```python
from build123d import *

# Parameters (mm, degrees)
SKETCH1_R           = 24
SKETCH1_R_2         = 17.8
BOSS_EXTRUDE1_DEPTH = 3.05
SKETCH2_R           = 23.3
SKETCH2_R_2         = 19
CUT_EXTRUDE1_DEPTH  = 0.8
SKETCH3_R           = 22.7
SKETCH3_R_2         = 19.6
BOSS_EXTRUDE2_DEPTH = 2.3


with BuildPart() as part:
    # Sketch1 → Boss-Extrude1 (new, symmetric)
    with BuildSketch(Plane.XY):
        Circle(SKETCH1_R)
        Circle(SKETCH1_R_2, mode=Mode.SUBTRACT)
    extrude(amount=BOSS_EXTRUDE1_DEPTH, both=True)

    # Sketch2 → Cut-Extrude1 (cut)
    with BuildSketch(Plane.XY.offset(3.05)):
        Circle(SKETCH2_R)
        Circle(SKETCH2_R_2, mode=Mode.SUBTRACT)
    cut_extrude1 = extrude(amount=-CUT_EXTRUDE1_DEPTH, mode=Mode.SUBTRACT)

    # Sketch3 → Boss-Extrude2 (add)
    with BuildSketch(Plane.XY.offset(2.25)):
        Circle(SKETCH3_R)
        Circle(SKETCH3_R_2, mode=Mode.SUBTRACT)
    boss_extrude2 = extrude(amount=BOSS_EXTRUDE2_DEPTH)

    # Mirror1: Cut-Extrude1, Boss-Extrude2 across plane
    add(cut_extrude1.mirror(Plane.XY), mode=Mode.SUBTRACT)
    add(boss_extrude2.mirror(Plane.XY))


solid = part.part
```
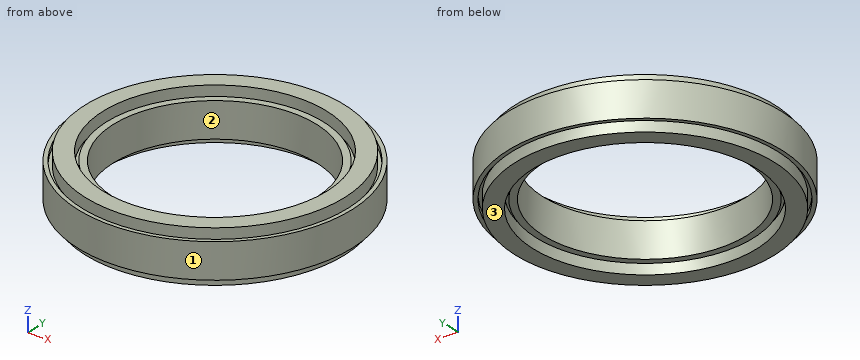
Here's how the part is built. I have some questions about the finished solid (model axes, mm). Face numbers are marked on the shaded views. Coordinates: 2 decimals unless noted, no trailing zeros. Write each loop counter-clockwise with the first axis right and the second up, starting at its lowest first coordinate (ties: lowest second). Pieces come first, ordered by that corner, then holes. Notation, with made-up numbers: (76, 23.25) -> (101, 23.25) arc R9 ccw to (101, 38.25) -> close; hole circle Ø3 at (-25, -23.75). An arc over 180 degrees is marked (long way). Use a Markdown table: item, result. Add a question column.
(1) Please list where these lines run through material, in increasing order: line 1 (Y direction, x = 0, z = -3.15); line 2 (X direction, y = 16, z = 2.5); line 3 (Y direction, x = 2.5, z = -3).
(2) I'm going to push flat-ended pins straight in: P1, Ø2, axis at y = -15, z = 0.5, coming from the -X side; P2, Ø1, axis at x = 15, z = 1.5, coming from the +Y side; P3, Ø14.5, axis at x = -3.5, y = -1.5, coming from the +Z side; P4, Ø5, axis at x = -12, z = -0.5, coming from the +Y side. Where does each tip first touch, or does it pass through?
(3) If we section it at A-A, the plane z = 1.25: Write out the boundary of the cut face in (x, y), and give its area (3 significant figures).
(4) We'd pull the mould along Y, two halves only. Please class the marked faces 1, 2 and 3: +Y half, -Y half, draft (parallel to the pull), parting line (faces both ways), or undercut.
Outcome:
| question | item | result |
|---|---|---|
| 1 | line 1 | y = -22.7 to -19.6, 19.6 to 22.7 |
| 1 | line 2 | x = -17.89 to -16.94, -16.1 to -11.32, -10.25 to -7.8, 7.8 to 10.25, 11.32 to 16.1, 16.94 to 17.89 |
| 1 | line 3 | y = -23.87 to -23.17, -22.56 to -19.44, -18.83 to -17.62, 17.62 to 18.83, 19.44 to 22.56, 23.17 to 23.87 |
| 2 | P1 | stops at x = -19.49 |
| 2 | P2 | stops at y = 19.12 |
| 2 | P3 | passes through |
| 2 | P4 | stops at y = 22.04 |
| 3 | outline | circle Ø48 at (0, 0); hole circle Ø35.6 at (0, 0) |
| 3 | area | 814 mm^2 |
| 4 | face 1 | parting line |
| 4 | face 2 | undercut |
| 4 | face 3 | draft |
